The drawing under review shows one solid part. Ordinate dimensions are in mm from its lowest x, y, z. A direction names the side the tool comes from. Coordinates: 2 decimals unless noted, no trailing zeros. Write each loop counter-clockwise with the first axis right and the second up, starting at its lowest first coordinate (ties: lowest second). Pieces come first, ordered by that corner, then holes.
Q1. Take a section at B-B (y = 2.75). Give the boundary of the cut face in (x, z) (1 decimal).
Q2. Machinability: for the marked faces 1 and 2, which of the approach directions +Z, -Z, +X, -X, +Y, -Y give a long, thin tool a straight path to every point of the face, cutting with its end or side? Answer none if there is none.
Q3. Take a section at C-C (x = 3.75). Give the boundary of the cut face in (y, z) (1 decimal).
Q4. Take a section at A-A (z = 28.5). Give the boundary of the cut face in (x, y) (1 decimal), and give its area (3 significant figures).
Q5. Insertion check: pin 1 (2 mm diameter, centred on x = 2.91, y = 3.18, fed in from +Z); pin 2 (1 mm diameter, centred on x = 4.5, z = 24, fed in from +Y); pin 3 (1 mm diameter, centred on y = 3.5, z = 9, fed in from -X). Each pin has a flat end and moves straight along its axis. Give the tip position at first contact, or say it passes through.
Q6. Take a section at D-D (z = 8). Give the boundary of the cut face in (x, y) (1 decimal).
Q7. For probe 1 along Z at (x, y) = (1.8, 2.25) (1 decimal); probe 2 along X at (y, z) = (2.75, 26); probe 3 along Y at (x, z) = (3.05, 12) (1 decimal), list the stretches that pass through material, from the lowest coordinate up.
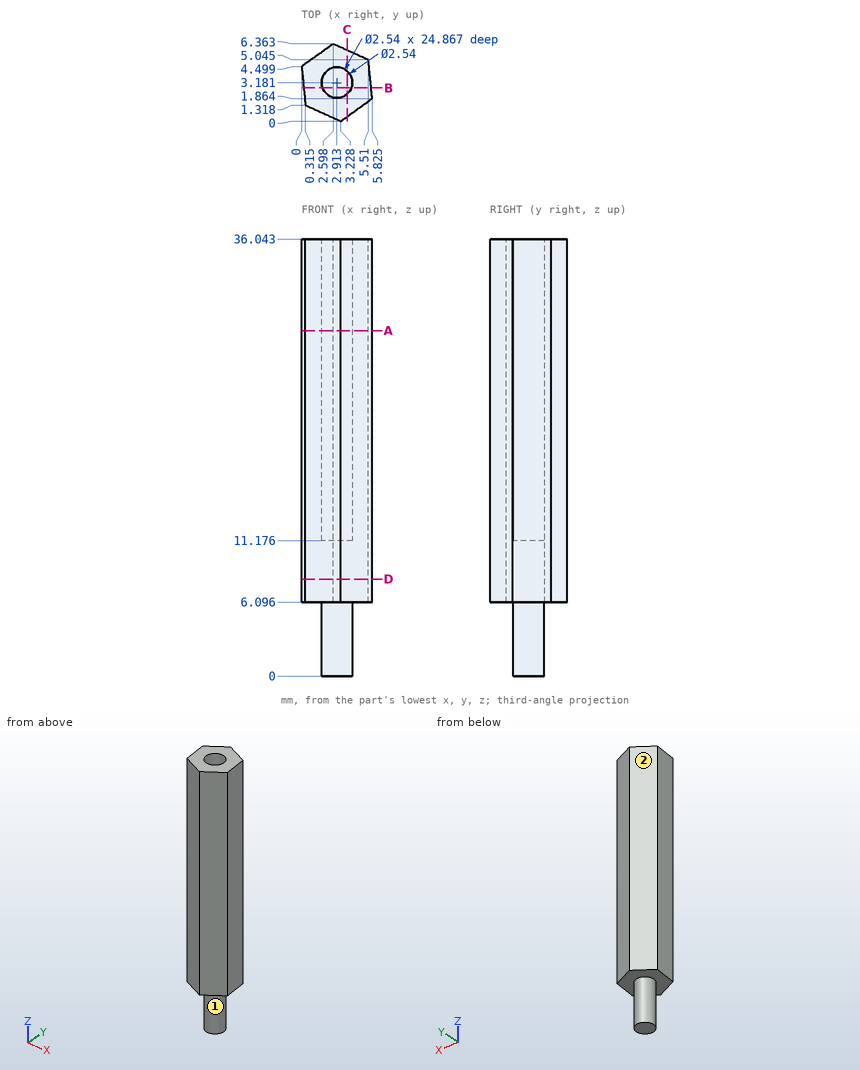
Response:
1. outline: (0.2, 6.1) - (1.7, 6.1) - (1.7, 0) - (4.1, 0) - (4.1, 6.1) - (5.7, 6.1) - (5.7, 36) - (4.1, 36) - (4.1, 11.2) - (1.7, 11.2) - (1.7, 36) - (0.2, 36) - close
2. face 1: -Z
2. face 2: +Z, -Z, -X, +Y
3. outline: (0.4, 6.1) - (2.2, 6.1) - (2.2, 0) - (4.1, 0) - (4.1, 6.1) - (5.8, 6.1) - (5.8, 36) - (4.1, 36) - (4.1, 11.2) - (2.2, 11.2) - (2.2, 36) - (0.4, 36) - close
4. outline: (0, 4.5) - (0.3, 1.3) - (3.2, 0) - (5.8, 1.9) - (5.5, 5) - (2.6, 6.4) - close; hole circle Ø2.5 at (2.9, 3.2)
4. area: 21.5 mm2
5. pin 1: stops at z = 11.18
5. pin 2: stops at y = 5.73
5. pin 3: stops at x = 0.05
6. outline: (0, 4.5) - (0.3, 1.3) - (3.2, 0) - (5.8, 1.9) - (5.5, 5) - (2.6, 6.4) - close
7. probe 1: z = 6.1 to 36
7. probe 2: x = 0.17 to 1.72, 4.11 to 5.74
7. probe 3: y = 0.1 to 1.9, 4.4 to 6.2
